Input: part model. Units: mm. Frame: model coordinates. A direction names the side the tool comes from. Give positions to 0.01 mm unless a question says otherwise; leave off trailing zeros. Loops run counter-clockwise (first coordinate to the right, second up) from the corner with the lowest first, then second, coordinate; pieces in that order, holes last. Notation, with made-up numbers: M 5,87 L 32,87 A22 cw 32,100 Z; hole C 85,-15.75 d1. An arc over 180 degrees is marked long. Answer as a JSON object with one key per item and string values. Group by question number.
1) Draft query along X for faces 4 (the cylindrical face through (9.26, -0.43, -7.26)), 5 (the flat face through (-10.05, -10, 4)), 6 (the flat face through (0, -13, -11.91)), 7 (the cylindrical face through (11.62, -11.5, -13.46)). Return one class per face: +X half, -X half, draft (parallel to the pull), parting line (faces both ways), or undercut.
2) Section query B-B on y = -4.5. Return loops of the section in (x, z).
3) First-contact query: P1, Ø2, axis at x = -1, y = -13.5, coming from the +Z side; P2, Ø3, axis at x = 0, z = 6.78, coming from the -Y side; P3, Ø2, axis at x = 2.5, y = 4, coming from the -Z side. Flat tips, straight axial feed; report the tip coordinate or a pass-through.
4) Section query D-D on z = 9.75. Return loops of the section in (x, y), plus the area to 3 significant figures.
5) Ray query, L1, parallel to Z at x = 5.1, y = -8.9; L2, parallel to X at y = -12.25, z = 8; L3, parallel to X at y = -1, z = -7.5. Return the intervals inside material, ascending.
6) Section query A-A on x = -5.1. Return loops of the section in (y, z), plus the area to 3 significant figures.
7) Section query C-C on x = 0. Return loops of the section in (y, z).
8) Access query for faces 1 (the flat face through (1.4, 3.09, 7.76)), 2 (the cylindrical face through (-6.87, -4.21, -5.94)), 3 (the flat face through (1.1, -4, -11)). Directions: +Z, -Z, +X, -X, +Y, -Y. A direction counts if a zero-diameter tool reaches every point of the face in a straight line with its end or side. Return the directions, or none.
Autodesk Inventor part; units mm, degrees
ref_plane "Work Plane1" through (0, 2, 0) normal (0, 1, 0) x (1, 0, 0)
ref_plane "YZ Plane" through (0, 0, 0) normal (1, 0, 0) x (0, 1, 0)
ref_plane "XZ Plane" through (0, 0, 0) normal (0, 1, 0) x (-1, 0, 0)
sketch "Sketch1" plane through (0, 0, 0) normal (0, 1, 0) x (-1, 0, 0)
  line L0 (12.05, 13.9095) -> (-12.05, 13.9095)
  line L1 (-12.05, 13.9095) -> (-12.05, -13.9095)
  line L2 (-12.05, -13.9095) -> (12.05, -13.9095)
  line L3 (12.05, -13.9095) -> (12.05, 13.9095)
  point P0 (0, 0)
  dimension "d0" = 24.1
  dimension "d1" = 12.05
  dimension "d2" = 27.819
  dimension "d3" = 13.9095
extrude "Extrusion1" add sketch "Sketch1" against normal blind 13.3
sketch "Sketch2" plane through (0, -13.3, 0) normal (0, -1, 0) x (1, 0, 0)
  line L0 (10.05, 13.9095) -> (-10.05, 13.9095)
  line L1 (-10.05, 13.9095) -> (-10.05, -11.9095)
  line L2 (-10.05, -11.9095) -> (10.05, -11.9095)
  line L3 (10.05, -11.9095) -> (10.05, 13.9095)
  line L4 (12.05, 13.9095) -> (-12.05, 13.9095)
  line L5 (12.05, -13.9095) -> (12.05, 13.9095)
  line L6 (-12.05, 13.9095) -> (-12.05, -13.9095)
  line L7 (-12.05, -13.9095) -> (12.05, -13.9095)
  point P0 (0, 0)
  dimension "d6" = 2
  dimension "d7" = 2
  dimension "d8" = 2
extrude "Extrusion2" cut sketch "Sketch2" against normal blind 10.8 contours L3 L2 L1 L0
sketch "Sketch3" plane through (0, 0, 0) normal (0, 1, 0) x (1, 0, 0)
  line L0 (-12.05, 5.7095) -> (12.05, 5.7095)
  line L1 (12.05, 5.7095) -> (12.05, 13.9095)
  line L2 (12.05, 13.9095) -> (-12.05, 13.9095)
  line L3 (-12.05, 13.9095) -> (-12.05, 5.7095)
  point P0 (0, 0)
  dimension "d11" = 8.2
extrude "Extrusion3" cut sketch "Sketch3" against normal blind 10.3
sketch "Sketch4" plane through (0, -10.3, 0) normal (0, 1, 0) x (1, 0, 0)
  line L0 (-1.1, 5.7095) -> (-12.05, 5.7095)
  line L1 (-12.05, 5.7095) -> (-12.05, 13.9095)
  line L2 (-12.05, 13.9095) -> (-1.1, 13.9095)
  line L3 (-1.1, 13.9095) -> (-1.1, 5.7095)
  point P0 (0, 0)
  dimension "d14" = 10.95
extrude "Extrusion4" add sketch "Sketch4" along normal blind 2
mirror "Mirror1" about plane through (0, 0, 0) normal (1, 0, 0) of "Extrusion4"
sketch "Sketch6" plane through (0, -13.3, 0) normal (0, -1, 0) x (1, 0, 0)
  line L0 (-12.05, -5.7095) -> (12.05, -5.7095)
  line L1 (12.05, -5.7095) -> (12.05, -13.9095)
  line L2 (12.05, -13.9095) -> (-12.05, -13.9095)
  line L3 (-12.05, -13.9095) -> (-12.05, -5.7095)
  point P0 (0, 0)
extrude "Extrusion6" add sketch "Sketch6" along normal blind 2
sketch "Sketch7" plane through (12.05, 0, -5.7095) normal (0, 0, -1) x (-1, 0, 0)
  line L0 (0, 0) -> (10.95, 0)
  line L1 (10.95, 0) -> (10.95, -8.3)
  line L2 (10.95, -8.3) -> (0, -8.3)
  line L3 (0, -8.3) -> (0, 0)
  point P0 (12.05, 0)
extrude "Extrusion7" add sketch "Sketch7" along normal blind 2
mirror "Mirror3" about plane through (0, 0, 0) normal (1, 0, 0) of "Extrusion7"
sketch "Sketch8" plane through (1.1, -8.3, -13.9095) normal (0, 1, 0) x (1, 0, 0)
  circle A0 centre (4, -4.719) radius 2.25
  line L0 (0, -8.2) -> (8.95, -8.2)
  line L1 (8.95, -27.819) -> (8.95, -8.2)
  line L2 (10.95, -27.819) -> (10.95, -6.2)
  line L3 (8.95, -2) -> (0, -2)
  point P0 (-1.1, -13.9095)
  dimension "d24" = 4.5
  dimension "d29" = 6.95
  dimension "d30" = 2.719
extrude "Extrusion8" cut sketch "Sketch8" against normal through all
mirror "Mirror4" about plane through (0, 0, 0) normal (1, 0, 0) of "Extrusion8"
sketch "Sketch9" plane through (0, 0, 0) normal (0, 1, 0) x (1, 0, 0)
  circle A0 centre (0, -6.7795) radius 1.15
  line L0 (-12.05, -13.9095) -> (12.05, -13.9095)
  circle A1 centre (0, -6.7795) radius 2.25
  point P0 (0, 0)
  dimension "d31" = 7.13
  dimension "d32" = 2.3
  dimension "d33" = 4.5
extrude "Extrusion9" add sketch "Sketch9" along normal blind 6.1
sketch "Sketch10" plane through (0, 6.1, 6.7795) normal (0, 1, 0) x (1, 0, 0)
  circle A0 centre (0, 0) radius 1.15
  arc A1 (-0.942, -0.6596) -> (0.942, -0.6596) centre (0, 0) ccw
  circle A2 centre (0, 0) radius 2.25
  arc A3 (-1.8431, -1.2905) -> (1.8431, -1.2905) centre (0, 0) ccw
  line L0 (0, 0) -> (-0.8052, 0)
  line L1 (0, 0) -> (0.4727, 0)
  line L2 (0, 0) -> (-0.942, -0.6596)
  line L3 (0, 0) -> (0.942, -0.6596)
  line L4 (-1.8431, -1.2905) -> (-0.942, -0.6596)
  line L5 (0.942, -0.6596) -> (1.8431, -1.2905)
  point P0 (0, 6.7795)
  dimension "d36" = 35
  dimension "d37" = 35
extrude "Extrusion10" cut sketch "Sketch10" against normal up to surface (6.1 mm away) contours A0 L5 A2 L4 picked at (-0.2694, -1.8509)
sketch "Sketch11" plane through (0, 0, 0) normal (0, 1, 0) x (1, 0, 0)
  line L0 (1.1, 5.7095) -> (-1.1, 5.7095)
  line L1 (-1.1, 5.7095) -> (-1.1, 7.7095)
  line L2 (-1.1, 7.7095) -> (-12.05, 7.7095)
  line L3 (-12.05, 7.7095) -> (-12.05, -13.9095)
  line L4 (-12.05, -13.9095) -> (12.05, -13.9095)
  line L5 (12.05, -13.9095) -> (12.05, 7.7095)
  line L6 (1.1, 7.7095) -> (12.05, 7.7095)
  line L7 (1.1, 5.7095) -> (1.1, 7.7095)
  arc A0 (0.942, -7.4391) -> (-0.942, -7.4391) centre (0, -6.7795) ccw
  line L8 (-0.942, -7.4391) -> (-1.8431, -8.07)
  arc A1 (1.8431, -8.07) -> (-1.8431, -8.07) centre (0, -6.7795) ccw
  line L9 (1.8431, -8.07) -> (0.942, -7.4391)
  circle A2 centre (0, -6.7795) radius 1.15
  point P0 (0, 0)
extrude "Extrusion11" cut sketch "Sketch11" against normal through all contours A2 A0
fillet "Fillet1" radius 2 1 edges at (0, 0, 4.5295)
fillet "Fillet2" radius 1.5 10 edges at (12.05, 0, 3.1) (-12.05, 0, 3.1) (6.575, 0, -7.7095) (-6.575, 0, -7.7095) (12.05, -4.15, -7.7095) (12.05, -8.3, -10.8095) (12.05, -11.8, -13.9095) (-12.05, -11.8, -13.9095) (-12.05, -8.3, -10.8095) (-12.05, -4.15, -7.7095)
sketch "Sketch12" plane through (0, -8.3, 0) normal (0, 1, 0) x (1, 0, 0)
  arc A0 (-3.4061, 7.7095) -> (-6.7939, 7.7095) centre (-5.1, 9.1905) ccw
  arc A1 (6.7939, 7.7095) -> (3.4061, 7.7095) centre (5.1, 9.1905) ccw
  circle A2 centre (-5.1, 9.1905) radius 2.25
  circle A3 centre (5.1, 9.1905) radius 2.25
  point P0 (0, 0)
extrude "Extrusion12" cut sketch "Sketch12" along normal through all both and the other way through all
sketch "Sketch13" plane through (0, -8.3, 0) normal (0, 1, 0) x (1, 0, 0)
  arc A0 (-3.4061, 7.7095) -> (-6.7939, 7.7095) centre (-5.1, 9.1905) ccw
  circle A1 centre (-5.1, 9.1905) radius 3.7
  arc A2 (6.7939, 7.7095) -> (3.4061, 7.7095) centre (5.1, 9.1905) ccw
  circle A3 centre (5.1, 9.1905) radius 3.7
  point P0 (0, 0)
  dimension "d46" = 7.4
  dimension "d47" = 7.4
extrude "Extrusion13" cut sketch "Sketch13" along normal through all
sketch "Sketch14" plane through (-10.05, -13.3, -5.7095) normal (0, 0, 1) x (1, 0, 0)
  line L0 (-2, 0) -> (22.1, 0)
  line L1 (22.1, 0) -> (22.1, -2)
  line L2 (22.1, -2) -> (-2, -2)
  line L3 (-2, -2) -> (-2, 0)
  point P0 (10.05, 13.3)
extrude "Extrusion14" cut sketch "Sketch14" along normal through all both and the other way through all
sketch "Sketch16" plane through (0, -13.3, 0) normal (0, -1, 0) x (1, 0, 0)
  line L0 (12.05, -12.4095) -> (12.05, 13.9095)
  line L1 (12.05, 13.9095) -> (10.05, 13.9095)
  line L2 (10.05, 13.9095) -> (10.05, -11.9095)
  line L3 (10.05, -11.9095) -> (-10.05, -11.9095)
  line L4 (-10.05, -11.9095) -> (-10.05, 13.9095)
  line L5 (-10.05, 13.9095) -> (-12.05, 13.9095)
  line L6 (-12.05, 13.9095) -> (-12.05, -12.4095)
  arc A0 (-12.05, -12.4095) -> (-10.55, -13.9095) centre (-10.55, -12.4095) ccw
  line L7 (10.55, -13.9095) -> (-10.55, -13.9095)
  arc A1 (10.55, -13.9095) -> (12.05, -12.4095) centre (10.55, -12.4095) ccw
  point P0 (0, 0)
extrude "Extrusion16" add sketch "Sketch16" along normal blind 1
sketch "Sketch17" plane through (0, -2.5, 0) normal (0, -1, 0) x (1, 0, 0)
  line L0 (10.05, -3.0905) -> (3.75, -3.0905)
  line L1 (3.75, -3.0905) -> (3.75, 13.9095)
  line L2 (3.75, 13.9095) -> (10.05, 13.9095)
  line L3 (10.05, 13.9095) -> (10.05, -3.0905)
  line L4 (-3.75, -3.0905) -> (-10.05, -3.0905)
  line L5 (-10.05, -3.0905) -> (-10.05, 13.9095)
  line L6 (-10.05, 13.9095) -> (-3.75, 13.9095)
  line L7 (-3.75, 13.9095) -> (-3.75, -3.0905)
  point P0 (0, 0)
  dimension "d57" = 7.5
  dimension "d58" = 6.3
  dimension "d59" = 17
extrude "Extrusion17" add sketch "Sketch17" along normal blind 1
sketch "Sketch18" plane through (0, -10.3, 0) normal (0, 1, 0) x (1, 0, 0)
  arc A0 (2.9083, 6.2095) -> (7.2917, 6.2095) centre (5.1, 9.1905) ccw
  arc A1 (-7.2917, 6.2095) -> (-2.9083, 6.2095) centre (-5.1, 9.1905) ccw
  line L0 (-1.1, 13.9095) -> (1.1, 13.9095)
  line L1 (1.1, 13.9095) -> (1.1, 5.7095)
  line L2 (1.1, 5.7095) -> (-1.1, 5.7095)
  line L3 (-1.1, 5.7095) -> (-1.1, 13.9095)
  point P0 (0, 0)
  point P1 (-1.7093, 7.7095)
extrude "Extrusion18" add sketch "Sketch18" along normal up to surface (10.3 mm away)
fillet "Fillet3" radius 2 1 edges at (0, 0, -13.9095)
sketch "Sketch19" plane through (0, 6.1, 0) normal (0, 1, 0) x (1, 0, 0)
  arc A0 (0.942, -7.4391) -> (-0.942, -7.4391) centre (0, -6.7795) ccw
  circle A1 centre (0, -6.7795) radius 1.225
  point P0 (0, 0)
  dimension "d65" = 2.45
extrude "Extrusion19" cut sketch "Sketch19" against normal up to surface (6.1 mm away)
sketch "Sketch20" plane through (0, 6.1, 0) normal (0, 1, 0) x (1, 0, 0)
  arc A0 (1.0035, -7.4821) -> (-1.0035, -7.4821) centre (0, -6.7795) ccw
  line L0 (1.0035, -7.4821) -> (1.8431, -8.07)
  arc A1 (1.8431, -8.07) -> (-1.8431, -8.07) centre (0, -6.7795) ccw
  line L1 (-1.8431, -8.07) -> (-1.0035, -7.4821)
  point P0 (0, 0)
extrude "Extrusion20" [suppressed]
ref_plane "Work Plane1" through (0, 2, 0) normal (0, 1, 0) x (1, 0, 0)
sketch "Sketch22" plane through (0, -14.3, 0) normal (0, -1, 0) x (1, 0, 0)
  line L0 (12.05, -12.4095) -> (12.05, 13.9095)
  line L1 (12.05, 13.9095) -> (10.05, 13.9095)
  line L2 (10.05, 13.9095) -> (10.05, -11.9095)
  line L3 (10.05, -11.9095) -> (-10.05, -11.9095)
  line L4 (-10.05, -11.9095) -> (-10.05, 13.9095)
  line L5 (-10.05, 13.9095) -> (-12.05, 13.9095)
  line L6 (-12.05, 13.9095) -> (-12.05, -12.4095)
  arc A0 (-12.05, -12.4095) -> (-10.55, -13.9095) centre (-10.55, -12.4095) ccw
  line L7 (-10.55, -13.9095) -> (10.55, -13.9095)
  arc A1 (10.55, -13.9095) -> (12.05, -12.4095) centre (10.55, -12.4095) ccw
  point P0 (0, 0)
extrude "Extrusion22" add sketch "Sketch22" along normal blind 0.5
equation "\"d37\" = d36"
properties part number "cover_dis"
Output:
{
 "1": {"face 4": "draft", "face 5": "undercut", "face 6": "undercut", "face 7": "+X half"},
 "2": {"outline": "M -12.05,-6.21 A1.5 ccw -10.55,-7.71 L -8.49,-7.71 A3.7 cw -6.35,-5.71 L -10.05,-5.71 L -10.05,13.91 L -12.05,13.91 Z; M -3.85,-5.71 A3.7 cw -1.71,-7.71 L -1.1,-7.71 L -1.1,-13.91 L 1.1,-13.91 L 1.1,-7.71 L 1.71,-7.71 A3.7 cw 3.85,-5.71 Z; M 6.35,-5.71 A3.7 cw 8.49,-7.71 L 10.55,-7.71 A1.5 ccw 12.05,-6.21 L 12.05,13.91 L 10.05,13.91 L 10.05,-5.71 Z"},
 "3": {"P1": "stops at z = -11.91", "P2": "stops at y = -2.5", "P3": "stops at z = 5.1"},
 "4": {"outline": "M -12.05,-14.8 L -10.05,-14.8 L -10.05,-3.5 L -3.75,-3.5 L -3.75,-2.5 L 3.75,-2.5 L 3.75,-3.5 L 10.05,-3.5 L 10.05,-14.8 L 12.05,-14.8 L 12.05,-1.5 A1.5 ccw 10.55,0 L -10.55,0 A1.5 ccw -12.05,-1.5 Z", "area": "121 mm^2"},
 "5": {"L1": "z = -13.91 to -11.44, -6.94 to -5.71", "L2": "x = -12.05 to -10.05, 10.05 to 12.05", "L3": "x = -11.13 to -8.39, -1.81 to 1.81, 8.39 to 11.13"},
 "6": {"outline": "M -14.8,-13.91 L -8.3,-13.91 L -8.3,-11.44 L -10.3,-11.44 L -10.3,-11.91 L -14.8,-11.91 Z; M -10.3,-6.94 L -8.3,-6.94 L -8.3,-5.71 L -10.3,-5.71 Z; M -3.5,-3.09 L -2.5,-3.09 L -2.5,-5.49 L 0,-5.49 L 0,13.91 L -3.5,13.91 Z", "area": "81.9 mm^2"},
 "7": {"outline": "M -14.8,-13.91 L -2,-13.91 A2 ccw 0,-11.91 L 0,2.53 A2 cw 2,4.53 L 6.1,4.53 L 6.1,5.55 L 0,5.55 L 0,5.63 L -2.5,5.63 L -2.5,-5.71 L -10.3,-5.71 L -10.3,-11.91 L -14.8,-11.91 Z; M -2.5,7.93 L 0,7.93 L 0,13.91 L -2.5,13.91 Z"},
 "8": {"face 1": "+Z, +Y", "face 2": "-Z, +Y", "face 3": "-Z, +X, +Y"}
}
